Design review of the part built by this model. Coordinates are the model's own, in mm. Face numbers are marked on the shaded views. A direction names the side the tool comes from. Give positions to 0.01 mm unless a question says otherwise; leave off trailing zeros. Loops run counter-clockwise (first coordinate to the right, second up) from the corner with the lowest first, then second, coordinate; pieces in that order, holes last. Notation, with made-up numbers: (76.5, -14) -> (106.5, -14) arc R21 cw to (106.5, 14) -> close; hole circle Ø3 at (25, -16). An arc over 180 degrees is marked (long way). Answer as CSV lines item,"result".
from build123d import *

# Parameters (mm, degrees)
SKETCH1_W           = 30
SKETCH1_H           = 30
BOSS_EXTRUDE1_DEPTH = 20
SKETCH2_R           = 3
SKETCH2_R_2         = 2.53
CUT_EXTRUDE1_DEPTH  = 40.05124838
SKETCH3_R           = 5
CUT_EXTRUDE2_DEPTH  = 15


with BuildPart() as part:
    # Sketch1 → Boss-Extrude1 (new body)
    with BuildSketch(Plane.XY):
        Rectangle(SKETCH1_W, SKETCH1_H)
    extrude(amount=BOSS_EXTRUDE1_DEPTH)

    # Sketch2 → Cut-Extrude1 (cut, through all)
    with BuildSketch(Plane(origin=(0, 15, 0), x_dir=(1, 0, 0), z_dir=(0, 1, 0))):
        with Locations(Location((-7.5, -10, 0), (0, 0, 270))):
            Circle(SKETCH2_R)
        with Locations(Location((7.5, -10, 0), (0, 0, 270))):
            Circle(SKETCH2_R_2)
    extrude(amount=-CUT_EXTRUDE1_DEPTH, mode=Mode.SUBTRACT)

    # Sketch3 → Cut-Extrude2 (cut)
    with BuildSketch(Plane(origin=(0, 15, 0), x_dir=(1, 0, 0), z_dir=(0, 1, 0))):
        with Locations(Location((-7.5, -10, 0), (0, 0, 270))):
            Circle(SKETCH3_R)
        with Locations(Location((7.5, -10, 0), (0, 0, 270))):
            Circle(SKETCH3_R)
    extrude(amount=-CUT_EXTRUDE2_DEPTH, mode=Mode.SUBTRACT)


solid = part.part
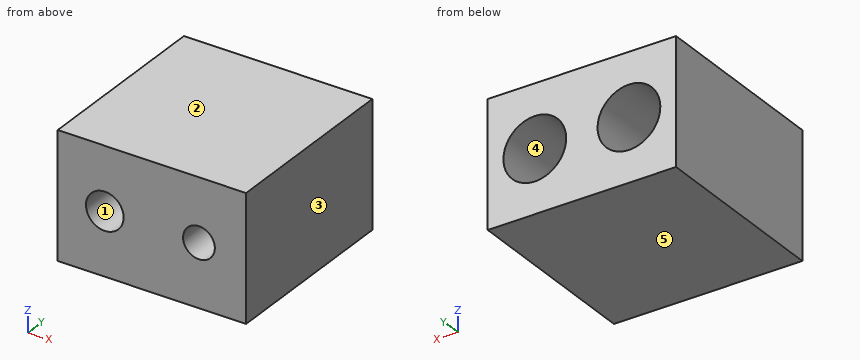
Q1. We need section B-B, the plane x = -7.5. State the section outline as (y, z) points.
Filled sheet:
outline,"(-15, 0) -> (15, 0) -> (15, 5) -> (0, 5) -> (0, 7) -> (-15, 7) -> close; (-15, 13) -> (0, 13) -> (0, 15) -> (15, 15) -> (15, 20) -> (-15, 20) -> close"
Q2. To check wall thickness, follow probe 1 along X at (y, z) = (-7.25, 10); probe 2 along X at (y, z) = (3.25, 10); probe 3 along Y at (x, z) = (6.5, 14). State the ranges of each line that lie inside material, in increasing order. Write a range as from..to.
Filled sheet:
probe 1,"x = -15..-10.5, -4.5..4.97, 10.03..15"
probe 2,"x = -15..-12.5, -2.5..2.5, 12.5..15"
probe 3,"y = -15..0"
Q3. Clearance check with flat-ended pins moving along their axes: pin 1 Ø8 at (x, z) = (7.5, 10) entering from +Y; pin 2 Ø4.5 at (x, z) = (7.5, 10) entering from -Y. State where each tip first meets the part, or that it passes through.
Filled sheet:
pin 1,"stops at y = 0"
pin 2,"passes through"
Q4. The part is to be moulded in two halves that separate along X. For the marked faces 1, 2 and 3, say which applies: pulls with the +X half, pulls with the -X half, needs draft (parallel to the pull), parting line crosses it, or undercut.
Filled sheet:
face 1,"undercut"
face 2,"needs draft"
face 3,"pulls with the +X half"
Q5. We need section D-D, the plane x = 7.5. State the section outline as (y, z) points, and give its area (3 significant figures).
Filled sheet:
outline,"(-15, 0) -> (15, 0) -> (15, 5) -> (0, 5) -> (0, 7.47) -> (-15, 7.47) -> close; (-15, 12.53) -> (0, 12.53) -> (0, 15) -> (15, 15) -> (15, 20) -> (-15, 20) -> close"
area,"374 mm^2"
Q6. We need section C-C, the plane y = -9.75. State the section outline as (x, z) points.
Filled sheet:
outline,"(-15, 0) -> (15, 0) -> (15, 20) -> (-15, 20) -> close; hole circle Ø6 at (-7.5, 10); hole circle Ø5.06 at (7.5, 10)"
Q7. For the marked faces 4 and 5, list the 3-axis set-ups (+Z, -Z, +X, -X, +Y, -Y) from which the entire face can be reached by the end or side of a thin tool; tool diameter is ignored.
Filled sheet:
face 4,"+Y"
face 5,"-Z, +X, -X, +Y, -Y"
Q8. We need section A-A, the plane z = 10. State the section outline as (x, y) points, and give its area (3 significant figures).
Filled sheet:
outline,"(-15, -15) -> (-10.5, -15) -> (-10.5, 0) -> (-12.5, 0) -> (-12.5, 15) -> (-15, 15) -> close; (-4.5, -15) -> (4.97, -15) -> (4.97, 0) -> (2.5, 0) -> (2.5, 15) -> (-2.5, 15) -> (-2.5, 0) -> (-4.5, 0) -> close; (10.03, -15) -> (15, -15) -> (15, 15) -> (12.5, 15) -> (12.5, 0) -> (10.03, 0) -> close"
area,"434 mm^2"
